Input: part model. Units: mm. Frame: model coordinates. A direction names the side the tool comes from. Coordinates: 2 decimals unless noted, no trailing zeros. Write each loop counter-clockwise with the first axis right and the second up, starting at its lowest first coordinate (ties: lowest second). Pieces come first, ordered by that corner, then holes. Notation, with made-up numbers: (55, -40) - (109, -40) arc R24 cw to (109, -23) - close; hole circle Ø3 at (-24.5, 13.25). An arc over 180 degrees is marked (long way). One line per question, with ' | ' between items. Start each with the question number.
1) Draft query along Z for faces 4 (the flat face through (-1, -32, 125)), 5 (the flat face through (0, -65, 121)), 6 (the flat face through (-1, -35, 120)). Return one class per face: released by +Z, released by -Z, zero draft, split by the parting line, or undercut.
2) Section query A-A on y = -19.5. Return loops of the section in (x, z), and give its area (3 significant figures).
3) Line query: line 1 (X direction, y = -7.5, z = 69.5); line 2 (Z direction, x = -34, y = -34); line 3 (Z direction, x = -98, y = -32). Output: solid intervals per line, ascending.
4) Reachability of faces 1 (the flat face through (-95, -35, -2)), 2 (the cylindrical face through (-97.53, -37.88, -81.57)), 3 (the flat face through (-100, -32, -2)) from +Z, -Z, +X, -X, +Y, -Y: full face, straight path, thin tool, end or side. Return the list, or none.
5) First-contact query: P1, Ø5, axis at x = -75, z = -100, coming from the +Y side; P2, Ø7, axis at x = -75, z = 100, coming from the +Y side. Flat tips, straight axial feed; report the tip coordinate or a pass-through.
6) Section query B-B on z = -33. Return loops of the section in (x, y).
7) Section query D-D on z = -90. Return loops of the section in (x, y).
8) Section query C-C on y = -32.5. Return loops of the section in (x, z), and give its area (3 significant figures).
```python
from build123d import *

# Parameters (mm, degrees)
F0_W     = 200
F0_H     = 250
F1_DEPTH = 5
F2_W     = 200
F2_H     = 250
F2_W_2   = 189.999994
F2_H_2   = 239.999994
F3_DEPTH = 60
F5_DEPTH = 5.001
F6_R     = 10
F7_DEPTH = 25


with BuildPart() as f1:
    # F0 (on Front) → F1 (new body)
    with BuildSketch(Plane.XZ):
        Rectangle(F0_W, F0_H)
    extrude(amount=F1_DEPTH)

    # F2 (on face) → F3 (join)
    with BuildSketch(Plane.XZ.offset(5)):
        Rectangle(F2_W, F2_H)
        Rectangle(F2_W_2, F2_H_2, mode=Mode.SUBTRACT)
    extrude(amount=F3_DEPTH)

    # F4 (on face) → F5 (cut, through all)
    with BuildSketch(Plane.XZ.offset(5)):
        with BuildLine():
            ThreePointArc((-74.999997, 96.999997), (-72.878677, 97.878677), (-71.999997, 99.999997))
            Line((-71.999997, 99.999997), (-74.999997, 99.999997))
            Line((-74.999997, 99.999997), (-74.999997, 96.999997))
        make_face()
        with BuildLine():
            Line((-74.999997, 99.999997), (-71.999997, 99.999997))
            ThreePointArc((-71.999997, 99.999997), (-77.121318, 102.121318), (-74.999997, 96.999997))
            Line((-74.999997, 96.999997), (-74.999997, 99.999997))
        make_face()
        with BuildLine():
            ThreePointArc((77.999997, 99.999997), (74.999997, 102.999997), (71.999997, 99.999997))
            Line((71.999997, 99.999997), (74.999997, 99.999997))
            Line((74.999997, 99.999997), (74.999997, 96.999997))
            ThreePointArc((74.999997, 96.999997), (77.121318, 97.878677), (77.999997, 99.999997))
        make_face()
        with BuildLine():
            Line((74.999997, 99.999997), (71.999997, 99.999997))
            ThreePointArc((71.999997, 99.999997), (72.878677, 97.878677), (74.999997, 96.999997))
            Line((74.999997, 96.999997), (74.999997, 99.999997))
        make_face()
        with BuildLine():
            ThreePointArc((77.999997, -99.999997), (77.121318, -97.878677), (74.999997, -96.999997))
            Line((74.999997, -96.999997), (74.999997, -99.999997))
            Line((74.999997, -99.999997), (71.999997, -99.999997))
            ThreePointArc((71.999997, -99.999997), (74.999997, -102.999997), (77.999997, -99.999997))
        make_face()
        with BuildLine():
            Line((74.999997, -99.999997), (74.999997, -96.999997))
            ThreePointArc((74.999997, -96.999997), (72.878677, -97.878677), (71.999997, -99.999997))
            Line((71.999997, -99.999997), (74.999997, -99.999997))
        make_face()
        with BuildLine():
            Line((-74.999997, -99.999997), (-74.999997, -96.999997))
            ThreePointArc((-74.999997, -96.999997), (-77.121318, -102.121318), (-71.999997, -99.999997))
            Line((-71.999997, -99.999997), (-74.999997, -99.999997))
        make_face()
        with BuildLine():
            ThreePointArc((-71.999997, -99.999997), (-72.878677, -97.878677), (-74.999997, -96.999997))
            Line((-74.999997, -96.999997), (-74.999997, -99.999997))
            Line((-74.999997, -99.999997), (-71.999997, -99.999997))
        make_face()
    extrude(amount=-F5_DEPTH, mode=Mode.SUBTRACT)

    # F6 (on face) → F7 (cut)
    with BuildSketch(Plane(origin=(-100, 0, 0), x_dir=(0, -1, 0), z_dir=(-1, 0, 0))):
        with Locations((32.5, -90)):
            Circle(F6_R)
    extrude(amount=-F7_DEPTH, mode=Mode.SUBTRACT)


solid = f1.part
```
Answer key:
1) face 4: released by +Z | face 5: zero draft | face 6: undercut
2) outline: (-100, -125) - (100, -125) - (100, 125) - (-100, 125) - close; hole (-95, -120) - (95, -120) - (95, 120) - (-95, 120) - close | area: 4,400 mm²
3) line 1: -100 to -95, 95 to 100 | line 2: -125 to -120, 120 to 125 | line 3: -125 to -99.99, -80.01 to 125
4) face 1: -Y | face 2: -X | face 3: +Z, -Z, -X, +Y, -Y
5) P1: through | P2: y = 0
6) outline: (-100, -65) - (-95, -65) - (-95, -5) - (95, -5) - (95, -65) - (100, -65) - (100, 0) - (-100, 0) - close
7) outline: (-100, -65) - (-95, -65) - (-95, -42.5) - (-100, -42.5) - close; (-100, -22.5) - (-95, -22.5) - (-95, -5) - (95, -5) - (95, -65) - (100, -65) - (100, 0) - (-100, 0) - close
8) outline: (-100, -125) - (100, -125) - (100, 125) - (-100, 125) - (-100, -80) - (-95, -80) - (-95, 120) - (95, 120) - (95, -120) - (-95, -120) - (-95, -100) - (-100, -100) - close | area: 4,300 mm²
